CAD build for the part. Positions are in the model's coordinates, mm. A direction names the side the tool comes from. Give positions to 0.01 mm unless a question says otherwise; leave off trailing zeros. Answer as CSV lines item,"result".
from build123d import *

# Parameters (mm, degrees)
F0_W     = 482.6
F0_H     = 482.6
F1_DEPTH = 609.6
F1_TAPER = -10
F2_SIZE  = 25.4


with BuildPart() as f1:
    # F0 (on Top) → F1 (new body)
    with BuildSketch(Plane.XY):
        Rectangle(F0_W, F0_H)
    extrude(amount=F1_DEPTH, taper=F1_TAPER)

    # F2
    f2_edges = [f1.edges().sort_by_distance(p)[0] for p in [
        (348.788927, 0, 609.6),
        (0, 348.788927, 609.6),
        (-348.788927, 0, 609.6),
        (0, -348.788927, 609.6),
    ]]
    chamfer(f2_edges, length=F2_SIZE)

    # F7 (on 3pt) → F8 (revolve, cut)
    with BuildSketch(Plane(origin=(0, 0, 0), x_dir=(-1, 0, 0), z_dir=(0, 1, 0))):
        with BuildLine():
            Line((-83.472505641, 508), (0, 508))
            Line((0, 508), (0, 609.6))
            Line((0, 609.6), (-266.7, 609.6))
            ThreePointArc((-266.7, 609.6), (-188.2280242177, 535.0998637348), (-83.472505641, 508))
        make_face()
    revolve(axis=Axis((0, 0, 445.9715634584), (0, 0, -1)), mode=Mode.SUBTRACT)


solid = f1.part
1) Drill centre lines: line 1 (Z direction, x = -49, y = -34.5); line 2 (X direction, y = -284.5, z = 433); line 3 (X direction, y = -18, z = 286). Where is each one in solid material? Low to high. Write a range as from..to.
Answer below:
line 1,"z = 0..508"
line 2,"x = -317.65..317.65"
line 3,"x = -291.73..291.73"
2) Flat gauge pins, fed straight in: pin 1 (2 mm diameter, centred on y = -143, z = 384.5, fed in from -X); pin 2 (3 mm diameter, centred on y = -139.5, z = 287, fed in from +X); pin 3 (1.5 mm diameter, centred on y = 40.5, z = 141, fed in from -X). Where does each tip first touch, or does it go through?
Answer below:
pin 1,"stops at x = -309.27"
pin 2,"stops at x = 292.17"
pin 3,"stops at x = -266.29"
3) Which spindle directions (+Z, -Z, +X, -X, +Y, -Y) get a long thin tool onto all of the face, cutting with end or side? Do faces 1 (the face through (-1, -1, 508)), 2 (the face through (189, -192, 609.6)). Say none if no direction does.
Answer below:
face 1,"+Z"
face 2,"+Z, +X, -X, +Y, -Y"
